```python
from build123d import *

# Parameters (mm, degrees)
F0_R     = 12.7
F0_R_2   = 1.5875
F0_R_3   = 2.413
F1_DEPTH = 1.9812
F2_R     = 4.953
F3_DEPTH = 2.8702
F4_R     = 2.9845
F5_DEPTH = 2.6924
F6_R     = 1.016
F7_DEPTH = 4.8524


with BuildPart() as f1:
    # F0 (on Front) → F1 (new body)
    with BuildSketch(Plane.XZ):
        Circle(F0_R)
        with Locations((0, -10.16)):
            Circle(F0_R_2, mode=Mode.SUBTRACT)
        with Locations((-9.271, 0)):
            Circle(F0_R_3, mode=Mode.SUBTRACT)
        with Locations((9.271, 0)):
            Circle(F0_R_3, mode=Mode.SUBTRACT)
        with Locations((0, 10.16)):
            Circle(F0_R_2, mode=Mode.SUBTRACT)
    extrude(amount=F1_DEPTH)

    # F2 (on face) → F3 (join)
    with BuildSketch(Plane(origin=(0, 0, 0), x_dir=(-1, 0, 0), z_dir=(0, 1, 0))):
        Circle(F2_R)
    extrude(amount=F3_DEPTH)

    # F4 (on face) → F5 (cut)
    with BuildSketch(Plane(origin=(0, 2.8702, 0), x_dir=(-1, 0, 0), z_dir=(0, 1, 0))):
        Circle(F4_R)
    extrude(amount=-F5_DEPTH, mode=Mode.SUBTRACT)

    # F6 (on face) → F7 (cut, through all)
    with BuildSketch(Plane.XZ.offset(1.9812)):
        Circle(F6_R)
    extrude(amount=-F7_DEPTH, mode=Mode.SUBTRACT)


solid = f1.part
```
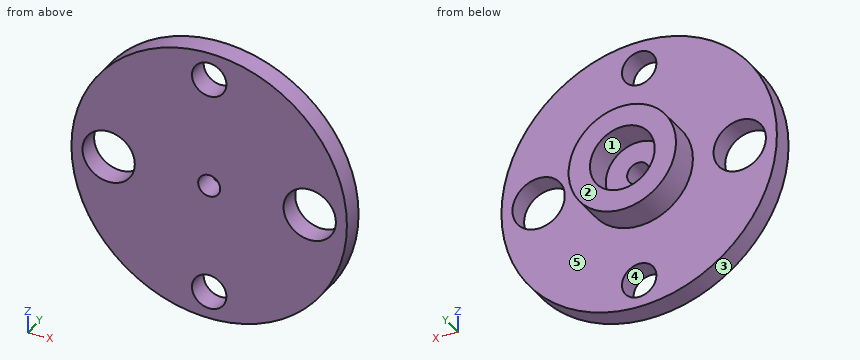
Geometry: final body of the model. Coordinates: model frame, mm. Face numbers are marked on the shaded views. A direction names the side the tool comes from. Round coordinates to 2 decimals unless told otherwise and drop trailing zeros. Order: outer loops, then holes, each group sorted by start corner. A loop starts at its lowest first (then second) coordinate and runs counter-clockwise, first axis right, second up. Notation, with made-up numbers: (-36, 36) -> (-18, 36) arc R34 ccw to (-18, 69) -> close; hole circle Ø3 at (-27.5, -31). An arc over 180 degrees is marked (long way). Use one line per item in the form item = value. Start each with the question number.
1. Pin query (flat end, axial travel): pin 1 Ø2.5 at (x, z) = (0, 0) entering from +Y; pin 2 Ø4 at (x, z) = (-9.271, 0) entering from +Y; pin 3 Ø4 at (x, z) = (7, -9) entering from +Y; pin 4 Ø1 at (x, y) = (-1.5, -1.5) entering from -Z. Return the tip coordinate at first contact, or that it passes through.
2. Cut plane B-B (z = 0). Return the cut outline in (x, y).
3. Line query: probe 1 along Z at (x, y) = (0, -1.05); probe 2 along Z at (x, y) = (0.5, -1.25); probe 3 along X at (y, z) = (-1.7, -11.5). Output: solid intervals per line, ascending.
4. Cut plane A-A (z = 10.16). Return the cut outline in (x, y).
5. Cut plane C-C (x = 0). Return the cut outline in (y, z).
6. Draft query along X for the marked faces 3, 4 and 5. Return one class per face: pulls with the +X half, pulls with the -X half, needs draft (parallel to the pull), parting line crosses it, or undercut.
7. Cut plane D-D (y = -1.4). Return the cut outline in (x, z) (1 decimal), then the cut area to 3 significant figures.
8. Reachability of the marked faces 1 and 2 from +Z, -Z, +X, -X, +Y, -Y: full face, straight path, thin tool, end or side. Return the list, or none.
Solution:
q1.pin_1 = 0.18
q1.pin_2 = through
q1.pin_3 = 0
q1.pin_4 = -12.66
q2.outline = (-12.7, -1.98) -> (-11.68, -1.98) -> (-11.68, 0) -> (-12.7, 0) -> close; (-6.86, -1.98) -> (-1.02, -1.98) -> (-1.02, 0.18) -> (-2.98, 0.18) -> (-2.98, 2.87) -> (-4.95, 2.87) -> (-4.95, 0) -> (-6.86, 0) -> close; (1.02, -1.98) -> (6.86, -1.98) -> (6.86, 0) -> (4.95, 0) -> (4.95, 2.87) -> (2.98, 2.87) -> (2.98, 0.18) -> (1.02, 0.18) -> close; (11.68, -1.98) -> (12.7, -1.98) -> (12.7, 0) -> (11.68, 0) -> close
q3.probe_1 = -12.7 to -11.75, -8.57 to -1.02, 1.02 to 8.57, 11.75 to 12.7
q3.probe_2 = -12.69 to -11.67, -8.65 to -0.88, 0.88 to 8.65, 11.67 to 12.69
q3.probe_3 = -5.39 to -0.85, 0.85 to 5.39
q4.outline = (-7.62, -1.98) -> (-1.59, -1.98) -> (-1.59, 0) -> (-7.62, 0) -> close; (1.59, -1.98) -> (7.62, -1.98) -> (7.62, 0) -> (1.59, 0) -> close
q5.outline = (-1.98, -12.7) -> (0, -12.7) -> (0, -11.75) -> (-1.98, -11.75) -> close; (-1.98, -8.57) -> (0, -8.57) -> (0, -4.95) -> (2.87, -4.95) -> (2.87, -2.98) -> (0.18, -2.98) -> (0.18, -1.02) -> (-1.98, -1.02) -> close; (-1.98, 1.02) -> (0.18, 1.02) -> (0.18, 2.98) -> (2.87, 2.98) -> (2.87, 4.95) -> (0, 4.95) -> (0, 8.57) -> (-1.98, 8.57) -> close; (-1.98, 11.75) -> (0, 11.75) -> (0, 12.7) -> (-1.98, 12.7) -> close
q6.face_3 = parting line crosses it
q6.face_4 = undercut
q6.face_5 = needs draft
q7.outline = circle Ø25.4 at (0, 0); hole circle Ø4.8 at (-9.3, 0); hole circle Ø3.2 at (0, -10.2); hole circle Ø3.2 at (0, 10.2); hole circle Ø2 at (0, 0); hole circle Ø4.8 at (9.3, 0)
q7.area = 451 mm^2
q8.face_1 = +Y
q8.face_2 = +Z, -Z, +X, -X, +Y
